from build123d import *

# Parameters (mm, degrees)
SKETCH1_R           = 46.355
BOSS_EXTRUDE1_DEPTH = 3.81
SKETCH2_R           = 33.02
SKETCH2_R_2         = 25.781
CUT_EXTRUDE1_DEPTH  = 2.54
CUT_EXTRUDE2_DEPTH  = 66.666491836
BOSS_EXTRUDE2_START = 12.7
SKETCH4_R           = 46.355
SKETCH4_R_2         = 44.45
BOSS_EXTRUDE2_DEPTH = 12.7


with BuildPart() as part:
    # Sketch1 → Boss-Extrude1 (new body)
    with BuildSketch(Plane.XY):
        with Locations(Location((0, 0, 0), (0, 0, 180))):
            Circle(SKETCH1_R)
    extrude(amount=BOSS_EXTRUDE1_DEPTH)

    # Sketch2 → Cut-Extrude1 (cut)
    with BuildSketch(Plane.XY.offset(3.81)):
        Circle(SKETCH2_R)
        Circle(SKETCH2_R_2, mode=Mode.SUBTRACT)
    extrude(amount=-CUT_EXTRUDE1_DEPTH, mode=Mode.SUBTRACT)

    # Sketch3 → Cut-Extrude2 (cut, through all)
    with BuildSketch(Plane.XY.offset(3.81)):
        with BuildLine():
            ThreePointArc((0, 33.02), (1.270941789, 32.995531621), (2.54, 32.922162748))
            Line((2.54, 32.922162748), (2.54, 38.002162748))
            Line((2.54, 38.002162748), (0, 38.002162748))
            Line((0, 38.002162748), (0, 33.02))
        make_face()
        with BuildLine():
            ThreePointArc((-2.54, 32.922162748), (-1.270941789, 32.995531621), (0, 33.02))
            Line((0, 33.02), (0, 38.002162748))
            Line((0, 38.002162748), (-2.54, 38.002162748))
            Line((-2.54, 38.002162748), (-2.54, 32.922162748))
        make_face()
        with BuildLine():
            Line((-38.002162748, -2.54), (-32.922162748, -2.54))
            ThreePointArc((-32.922162748, -2.54), (-33.02, 0), (-32.922162748, 2.54))
            Line((-32.922162748, 2.54), (-38.002162748, 2.54))
            Line((-38.002162748, 2.54), (-38.002162748, -2.54))
        make_face()
        with BuildLine():
            Line((2.54, -38.002162748), (2.54, -32.922162748))
            ThreePointArc((2.54, -32.922162748), (0, -33.02), (-2.54, -32.922162748))
            Line((-2.54, -32.922162748), (-2.54, -38.002162748))
            Line((-2.54, -38.002162748), (2.54, -38.002162748))
        make_face()
        with BuildLine():
            ThreePointArc((33.02, 0), (32.995531621, -1.270941789), (32.922162748, -2.54))
            Line((32.922162748, -2.54), (38.002162748, -2.54))
            Line((38.002162748, -2.54), (38.002162748, 2.54))
            Line((38.002162748, 2.54), (32.922162748, 2.54))
            ThreePointArc((32.922162748, 2.54), (32.995531621, 1.270941789), (33.02, 0))
        make_face()
    extrude(amount=-CUT_EXTRUDE2_DEPTH, mode=Mode.SUBTRACT)

    # Sketch4 → Boss-Extrude2 (add)
    with BuildSketch(Plane(origin=(0, 0, 0), x_dir=(-1, 0, 0), z_dir=(0, 0, -1)).offset(BOSS_EXTRUDE2_START)):
        Circle(SKETCH4_R)
        with Locations(Location((0, 0, 0), (0, 0, 180))):
            Circle(SKETCH4_R_2, mode=Mode.SUBTRACT)
    extrude(amount=-BOSS_EXTRUDE2_DEPTH)


solid = part.part
The listing builds one solid part. Answer for the finished solid, in the listing's coordinates (mm). A direction names the side the tool comes from. Round coordinates to 2 decimals unless told otherwise and drop trailing zeros. Write each loop counter-clockwise with the first axis right and the second up, starting at its lowest first coordinate (ties: lowest second). Pieces come first, ordered by that corner, then holes. Notation, with made-up numbers: (6, 24.25) - (56, 24.25) arc R11 ccw to (56, 33.25) - close; hole circle Ø9 at (39, 30). An arc over 180 degrees is marked (long way). Use one line per item in the form item = value. Start each with the question number.
Item 1: A cutting plane is placed at A-A (z = -7). Write down the section's boundary in (x, y) (3 decimals), plus the area to 3 significant figures.
Item 2: Find the intervals of material crossed by line 1 (Y direction, x = 0, z = -3) (3 decimals); line 2 (X direction, y = -13.5, z = 2); line 3 (Z direction, x = -3.5, y = -2), in increasing order. Write a range as [from, to].
Item 3: A cutting plane is placed at C-C (x = -13.5). Write down the section's boundary in (y, z).
Item 4: A cutting plane is placed at D-D (x = -31.5). Write down the section's boundary in (y, z), plus the area to 3 significant figures.
Item 5: Determine the mould class of faces 1 (the flat face through (0, 0, 3.81)), 2 (the cylindrical face through (-23.579, -23.116, 2.558)), 3 (the flat face through (35, 2.54, 2)) for opening direction Y: +Y half, -Y half, draft (parallel to the pull), parting line (faces both ways), or undercut.
Item 6: A tool of negligible diameter and unlimited length cuts with its end or side. For faces 4 (the flat face through (-38, -24, -12.7)), 5 (the cylindrical face through (-3.36, 25.56, 2.56)), 6 (the flat face through (38.002, 0, 2)), 7 (the flat face through (1, -1, 0)), from which of +Z, -Z, +X, -X, +Y, -Y can it reach the whole face along a straight path? Write none if from no direction.
Item 7: A cutting plane is placed at B-B (y = -9). Write down the section's boundary in (x, z).
Item 8: Flat-ended cylindrical pins translate along their axes: pin 1 Ø4 at (y, z) = (36, 1.5) entering from +X; pin 2 Ø4 at (x, z) = (-35, 2) entering from +Y; pin 3 Ø1 at (x, y) = (-12.5, -13.5) entering from -Z. Find the tip coordinate at first contact, or state that the pin passes through.
The answers:
q1.outline = circle Ø92.71 at (0, 0); hole circle Ø88.9 at (0, 0)
q1.area = 543 mm^2
q2.line_1 = [-46.355, -44.45], [44.45, 46.355]
q2.line_2 = [-44.35, -30.13], [-21.96, 21.96], [30.13, 44.35]
q2.line_3 = [0, 3.81]
q3.outline = (-44.35, -12.7) - (-42.35, -12.7) - (-42.35, 0) - (42.35, 0) - (42.35, -12.7) - (44.35, -12.7) - (44.35, 3.81) - (30.13, 3.81) - (30.13, 1.27) - (21.96, 1.27) - (21.96, 3.81) - (-21.96, 3.81) - (-21.96, 1.27) - (-30.13, 1.27) - (-30.13, 3.81) - (-44.35, 3.81) - close
q4.outline = (-34.01, -12.7) - (-31.36, -12.7) - (-31.36, 0) - (31.36, 0) - (31.36, -12.7) - (34.01, -12.7) - (34.01, 3.81) - (9.9, 3.81) - (9.9, 1.27) - (-9.9, 1.27) - (-9.9, 3.81) - (-34.01, 3.81) - close
q4.area = 276 mm^2
q5.face_1 = draft
q5.face_2 = undercut
q5.face_3 = undercut
q6.face_4 = -Z, +X, -X, +Y, -Y
q6.face_5 = +Z
q6.face_6 = +Z, -Z
q6.face_7 = -Z
q7.outline = (-45.47, -12.7) - (-43.53, -12.7) - (-43.53, 0) - (43.53, 0) - (43.53, -12.7) - (45.47, -12.7) - (45.47, 3.81) - (31.77, 3.81) - (31.77, 1.27) - (24.16, 1.27) - (24.16, 3.81) - (-24.16, 3.81) - (-24.16, 1.27) - (-31.77, 1.27) - (-31.77, 3.81) - (-45.47, 3.81) - close
q8.pin_1 = 31.51
q8.pin_2 = 32.55
q8.pin_3 = 0
